Design review of the part built by this model. Coordinates are the model's own, in mm. A direction names the side the tool comes from. Give positions to 0.01 mm unless a question says otherwise; leave off trailing zeros. Write each loop counter-clockwise with the first axis right and the second up, starting at its lowest first coordinate (ties: lowest second). Pieces come first, ordered by that corner, then holes.
```python
from build123d import *

# Parameters (mm, degrees)
PAD003_DEPTH  = 1.6
SKETCH011_W   = 1.3
SKETCH011_H   = 16
PAD004_DEPTH  = 2.25
SKETCH012_W   = 0.8
SKETCH012_H   = 0.65
SKETCH012_W_2 = 0.85
PAD005_DEPTH  = 15


with BuildPart() as part:
    # Sketch008 → Pad003 (new body)
    with BuildSketch(Plane.XY.offset(85)):
        with BuildLine():
            Line((30.57387, -6.02613), (30.57387, -27.02613))
            ThreePointArc((28, -29.6), (29.820001, -28.846131), (30.57387, -27.02613))
            Line((28, -29.6), (-28, -29.6))
            ThreePointArc((-30.57387, -27.02613), (-29.820001, -28.846131), (-28, -29.6))
            Line((-30.57387, -27.02613), (-30.57387, -6.02613))
            ThreePointArc((-30.57387, -6.02613), (-29.827263, -7.828603), (-28.02479, -8.575212))
            Line((-28.02479, -8.575212), (-26.12479, -8.575212))
            Line((-26.12479, -8.575212), (-26.12479, -13.175212))
            Line((-26.12479, -13.175212), (-16.47479, -13.175212))
            Line((-16.47479, -13.175212), (-16.47479, -22.375212))
            Line((-16.47479, -22.375212), (-4.47479, -22.375212))
            Line((-4.47479, -22.375212), (-4.47479, -13.175212))
            Line((-4.47479, -13.175212), (1.72521, -13.175212))
            Line((1.72521, -13.175212), (1.72521, -22.153704))
            Line((1.72521, -22.153704), (14.22521, -22.153704))
            Line((14.22521, -22.153704), (14.22521, -11.153704))
            Line((14.22521, -11.153704), (26.12521, -11.153704))
            Line((26.12521, -11.153704), (26.12521, -8.553704))
            Line((26.12521, -8.553704), (28.35521, -8.553704))
            ThreePointArc((28.35521, -8.553704), (29.940524, -7.707728), (30.57387, -6.02613))
        make_face()
    extrude(amount=PAD003_DEPTH)

    # Sketch011 → Pad004 (new body)
    with BuildSketch(Plane(origin=(0, 0, 85), x_dir=(1, 0, 0), z_dir=(0, 0, -1))):
        with Locations((-28.27479, 16.575212)):
            Rectangle(SKETCH011_W, SKETCH011_H)
        with Locations((28.27521, 16.553704)):
            Rectangle(SKETCH011_W, SKETCH011_H)
    extrude(amount=PAD004_DEPTH)

    # Sketch012 → Pad005 (new body)
    with BuildSketch(Plane(origin=(0, -8.553704, 85), x_dir=(-1, 0, 0), z_dir=(0, 1, 0))):
        with Locations((29.32479, -1.925)):
            Rectangle(SKETCH012_W, SKETCH012_H)
        with Locations((-29.35021, -1.925)):
            Rectangle(SKETCH012_W_2, SKETCH012_H)
    extrude(amount=-PAD005_DEPTH)


solid = part.part
```
(1) Consider section B-B, the plane y = -7.25. Give the boundary of the cut face in (x, z).
Resolved:
outline: (-30.57, 85) - (-30.26, 85) - (-30.26, 86.6) - (-30.57, 86.6) - close; (30.26, 85) - (30.57, 85) - (30.57, 86.6) - (30.26, 86.6) - close
(2) Mouldability with a two-part tool opening along X and no side actions: class faces 1 (the face through (-29.847, -7.809, 85.789)), 2 (the face through (28, -24.554, 84)), 3 (the face through (29.8, -28.866, 85.789)) as pulls with the +X half, pulls with the -X half, needs draft (parallel to the pull), parting line crosses it, or undercut.
Resolved:
face 1: undercut
face 2: needs draft
face 3: pulls with the +X half
(3) Consider section A-A, the plane y = -20.25. Give the boundary of the cut face in (x, z), then the cut area to 3 significant figures.
Resolved:
outline: (-30.57, 85) - (-28.92, 85) - (-28.92, 83.4) - (-29.72, 83.4) - (-29.72, 82.75) - (-27.62, 82.75) - (-27.62, 85) - (-16.47, 85) - (-16.47, 86.6) - (-30.57, 86.6) - close; (-4.47, 85) - (1.73, 85) - (1.73, 86.6) - (-4.47, 86.6) - close; (14.23, 85) - (27.63, 85) - (27.63, 82.75) - (29.78, 82.75) - (29.78, 83.4) - (28.93, 83.4) - (28.93, 85) - (30.57, 85) - (30.57, 86.6) - (14.23, 86.6) - close
area: 65.6 mm2
(4) Consider section C-C, the plane x = 13. Give the boundary of the cut face in (y, z), then the cut area to 3 significant figures.
Resolved:
outline: (-29.6, 85) - (-22.15, 85) - (-22.15, 86.6) - (-29.6, 86.6) - close
area: 11.9 mm2
(5) To check wall thickness, follow L1, parallel to X at y = -19.25, z = 84.85; L2, parallel to X at y = -18.25, z = 86.35; L3, parallel to X at y = -9.5, z = 85.8. State the ranges of each line that lie inside material, in increasing order.
Resolved:
L1: x = -28.92 to -27.62, 27.63 to 28.93
L2: x = -30.57 to -16.47, -4.47 to 1.73, 14.23 to 30.57
L3: x = -30.57 to -26.12, 26.13 to 30.57
(6) Tool access review of faces 4 (the face through (-28, -24.575, 84)), 5 (the face through (8, -22.154, 86)), 6 (the face through (27.625, -16, 84)), 7 (the face through (-27.9, -8.575, 84.7)), 8 (the face through (-29, -16, 82.75)): name each direction out of +Z, -Z, +X, -X, +Y, -Y from which nothing blocks a thin tool from reaching the whole face with its end or side.
Resolved:
face 4: -Z, +X, -X, -Y
face 5: +Z, -Z, +Y
face 6: -Z, +Y, -Y
face 7: -Z, +Y
face 8: -Z, +X, -X, +Y, -Y
(7) Clearance check with flat-ended pins moving along their axes: P1, Ø1.8, axis at y = -19.5, z = 84, coming from the +X side; P2, Ø7, axis at x = -7.5, y = -21.5, coming from the -Z side; P3, Ø0.7, axis at y = -16, z = 83, coming from the -X side; P4, Ø3, axis at x = -2, y = -10.5, coming from the -Z side. State where each tip first meets the part, or that it passes through.
Resolved:
P1: stops at x = 29.78
P2: stops at z = 85
P3: stops at x = -29.72
P4: passes through
(8) Consider section D-D, the plane y = -26. Give the boundary of the cut face in (x, z), then the cut area to 3 significant figures.
Resolved:
outline: (-30.57, 85) - (30.57, 85) - (30.57, 86.6) - (-30.57, 86.6) - close
area: 97.8 mm2
